The figure shows three views and two pictorial views of one solid part (mm, origin at its lowest corner). Answer the questions. A direction names the side the tool comes from. Give positions to 0.01 mm unless a question says otherwise; leave off trailing zeros. Order: outer loops, then holes, each group sorted by start corner. A loop starts at its lowest first (then second) coordinate and runs counter-clockwise, first axis right, second up. Notation, with made-up numbers: M 85,67 L 128,67 A14 cw 128,91 Z; hole C -13.5,-31 d11. An arc over 180 degrees is marked long. Write item = value, one per line. Start each with the question number.
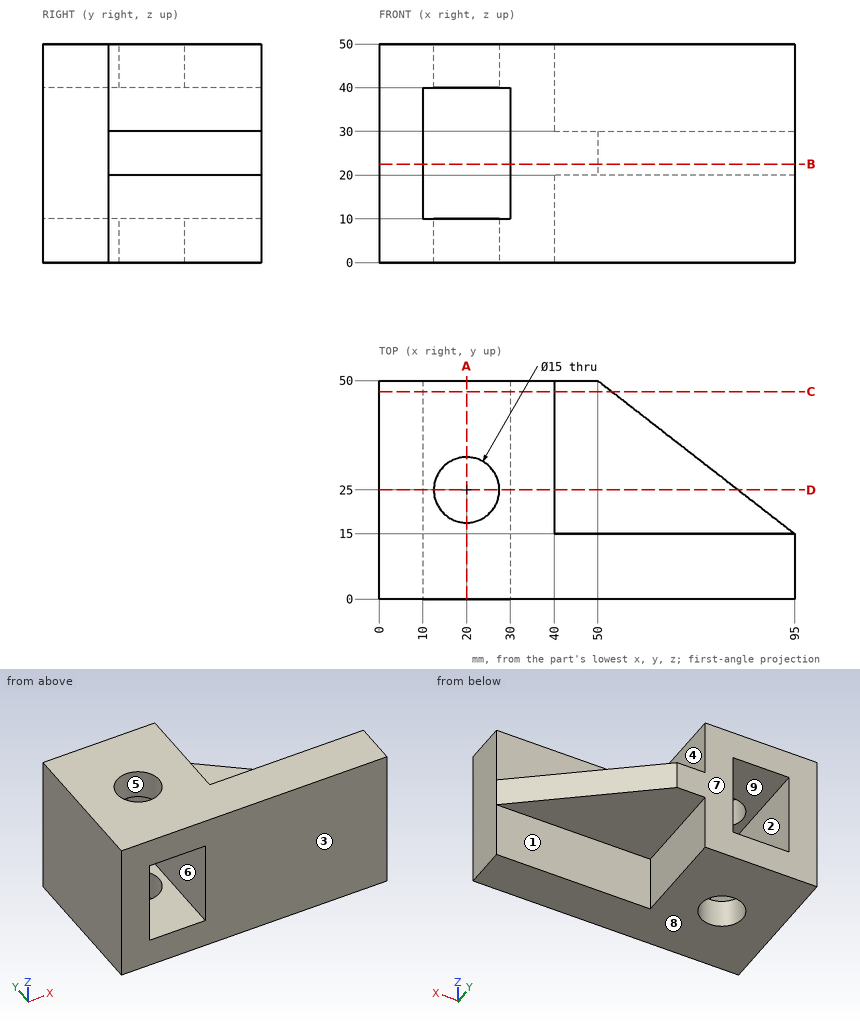
1) For the marked faces 1, 2, 3, 4 and 5, determine the directions among +Z, -Z, +X, -X, +Y, -Y from which every point of the face is accessible in a straight line to the end or side of a thin tool.
2) Each of these flat-tipped pins is pushed along its axis until it touches: P1, Ø6, axis at y = 20, z = 36, coming from the +X side; P2, Ø12, axis at y = 41, z = 19, coming from the +X side; P3, Ø9, axis at y = 26.5, z = 25.5, coming from the +X side. Where does it stop, or does it pass through?
3) Find the intervals of material crossed by probe 1 along Z at (x, y) = (24, 15); probe 2 along Y at (x, z) = (20, 44); probe 3 along X at (y, z) = (34, 30.5), in increasing order. Write a range as [from, to].
4) Find section B-B on z = 22.5. Determine the outline of the cut face in (x, y).
5) For a pull along Z with two mould halves and no side action, classify the marked faces 6, 7, 8 and 9 as pulls with the +Z half, pulls with the -Z half, needs draft (parallel to the pull), parting line crosses it, or undercut.
6) Find section A-A on x = 20. Determine the outline of the cut face in (y, z).
7) Find section D-D on y = 25. Determine the outline of the cut face in (x, z).
8) Find section C-C on y = 47.5. Determine the outline of the cut face in (x, z), plus the area to 3 significant figures.
Numbers:
q1.face_1 = -Z, +X, +Y
q1.face_2 = +Y, -Y
q1.face_3 = +Z, -Z, +X, -X, -Y
q1.face_4 = +Z, +X, +Y
q1.face_5 = +Z, -Z
q2.P1 = 40
q2.P2 = 69.18
q2.P3 = 86
q3.probe_1 = [0, 10], [40, 50]
q3.probe_2 = [0, 17.5], [32.5, 50]
q3.probe_3 = [0, 10], [30, 40]
q4.outline = M 0,0 L 10,0 L 10,50 L 0,50 Z; M 30,0 L 95,0 L 95,15 L 50,50 L 30,50 Z
q5.face_6 = undercut
q5.face_7 = needs draft
q5.face_8 = pulls with the -Z half
q5.face_9 = undercut
q6.outline = M 0,0 L 17.5,0 L 17.5,10 L 0,10 Z; M 0,40 L 17.5,40 L 17.5,50 L 0,50 Z; M 32.5,0 L 50,0 L 50,10 L 32.5,10 Z; M 32.5,40 L 50,40 L 50,50 L 32.5,50 Z
q7.outline = M 0,0 L 12.5,0 L 12.5,10 L 10,10 L 10,40 L 12.5,40 L 12.5,50 L 0,50 Z; M 27.5,0 L 40,0 L 40,20 L 82.14,20 L 82.14,30 L 40,30 L 40,50 L 27.5,50 L 27.5,40 L 30,40 L 30,10 L 27.5,10 Z
q8.outline = M 0,0 L 40,0 L 40,20 L 53.21,20 L 53.21,30 L 40,30 L 40,50 L 0,50 Z; hole M 10,10 L 30,10 L 30,40 L 10,40 Z
q8.area = 1,530 mm2
